Geometry: see drawing. Coordinates: mm, zero at the bounding-box minimum. A direction names the side the tool comes from. Give positions to 0.01 mm unless a question says otherwise; leave off trailing zeros. Write each loop counter-clockwise with the first axis right and the second up, starting at its lowest first coordinate (ties: lowest second). Pieces come first, ordered by that corner, then holes. Notation, with made-up numbers: (46, 57.5) -> (71, 57.5) arc R14 ccw to (71, 63.5) -> close; hole circle Ø6 at (-26.75, 41). An arc over 180 degrees is marked (long way). Answer as a JSON object with one key per item and string values. Group by question number.
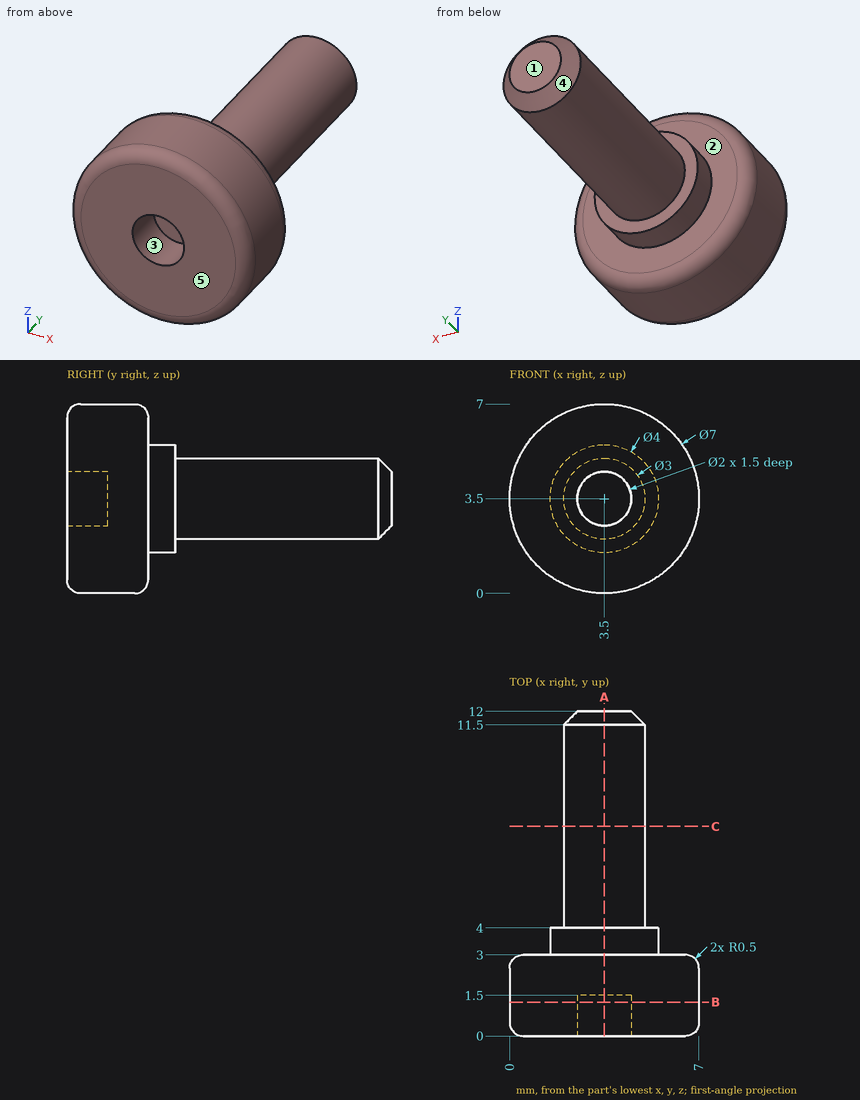
1. Mould query, pull axis X, two halves, no side actions, for the marked faces 3, 4 and 5. Classes: pulls with the +X half, pulls with the -X half, needs draft (parallel to the pull), parting line crosses it, or undercut.
2. Reachability of the marked faces 1 and 2 from +Z, -Z, +X, -X, +Y, -Y: full face, straight path, thin tool, end or side. Return the list, or none.
3. Section A-A (x = 3.5). Return the cut outline in (y, z).
4. Contact query for flat-ended pins moving along their axis: pin 1 Ø3 at (x, y) = (6, 2.5) entering from +Z; pin 2 Ø2 at (x, y) = (3, 10.5) entering from -Z; pin 3 Ø0.6 at (x, z) = (3.5, 4) entering from -Y. Output: stop coordinate, or through.
5. Line query: line 1 (X direction, y = 0.85, z = 3.5); line 2 (Y direction, x = 3, z = 3.5); line 3 (Y direction, x = 6.25, z = 3). Output: solid intervals per line, ascending.
6. Section C-C (y = 7.75). Return the cut outline in (x, z), plus the area to 3 significant figures.
7. Section B-B (y = 1.25). Return the cut outline in (x, z), plus the area to 3 significant figures.
Working result:
{
 "1": {"face 3": "undercut", "face 4": "parting line crosses it", "face 5": "needs draft"},
 "2": {"face 1": "+Z, -Z, +X, -X, +Y", "face 2": "+Y"},
 "3": {"outline": "(0, 0.5) arc R0.5 ccw to (0.5, 0) -> (2.5, 0) arc R0.5 ccw to (3, 0.5) -> (3, 1.5) -> (4, 1.5) -> (4, 2) -> (11.5, 2) -> (12, 2.5) -> (12, 4.5) -> (11.5, 5) -> (4, 5) -> (4, 5.5) -> (3, 5.5) -> (3, 6.5) arc R0.5 ccw to (2.5, 7) -> (0.5, 7) arc R0.5 ccw to (0, 6.5) -> (0, 4.5) -> (1.5, 4.5) -> (1.5, 2.5) -> (0, 2.5) -> close"},
 "4": {"pin 1": "stops at z = 6.85", "pin 2": "stops at z = 2", "pin 3": "stops at y = 1.5"},
 "5": {"line 1": "x = 0 to 2.5, 4.5 to 7", "line 2": "y = 1.5 to 12", "line 3": "y = 0 to 3"},
 "6": {"outline": "circle Ø3 at (3.5, 3.5)", "area": "7.07 mm^2"},
 "7": {"outline": "circle Ø7 at (3.5, 3.5); hole circle Ø2 at (3.5, 3.5)", "area": "35.3 mm^2"}
}
